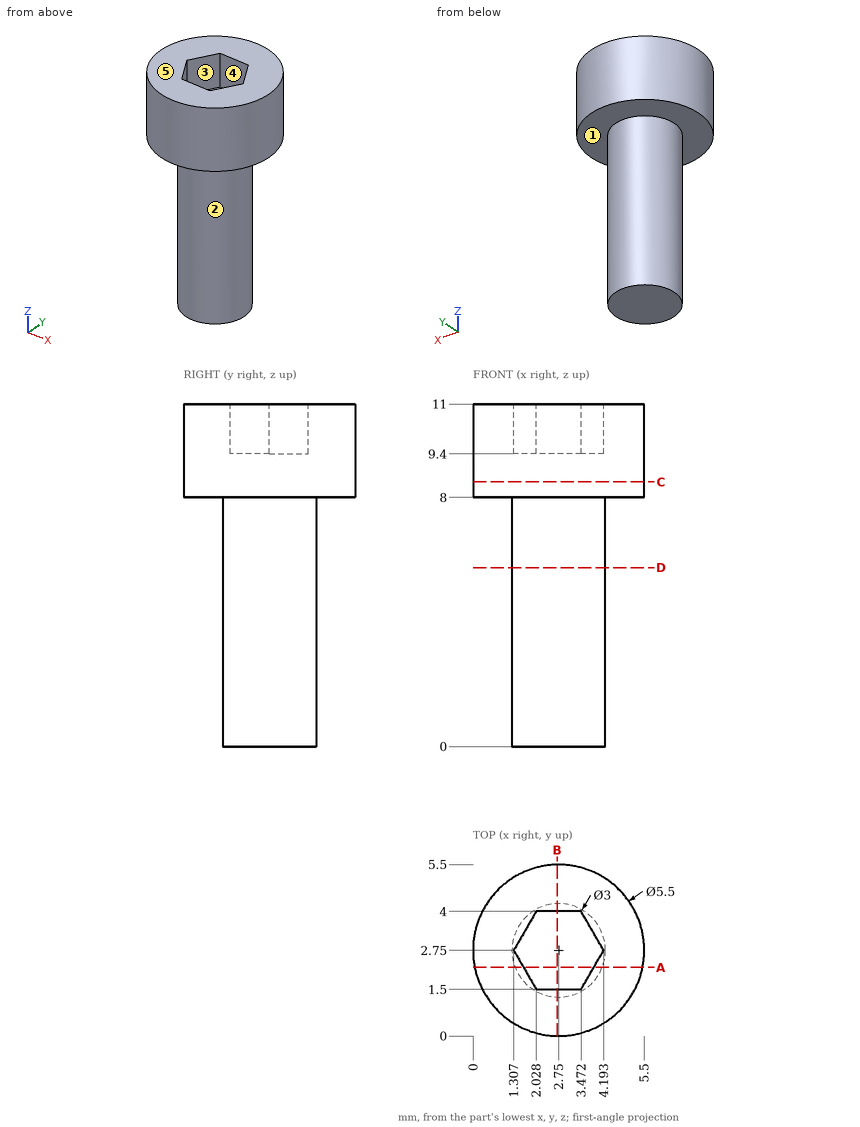
Verification items for this drawing (mm, ordinates from the low corner). A direction names the side the tool comes from. Coordinates: 2 decimals unless noted, no trailing zeros. Order: outer loops, then holes, each group sorted by start corner. A loop starts at its lowest first (then second) coordinate and runs counter-clockwise, first axis right, second up.
Q1. Sectioned sample at A-A on y = 2.2. Record the cut outline in (x, z) (1 decimal).
Reply:
outline: (0.1, 8) - (1.4, 8) - (1.4, 0) - (4.1, 0) - (4.1, 8) - (5.4, 8) - (5.4, 11) - (3.9, 11) - (3.9, 9.4) - (1.6, 9.4) - (1.6, 11) - (0.1, 11) - close
Q2. Tool access check on the marked faces 4 and 5. Record the directions out of +Z, -Z, +X, -X, +Y, -Y that give a thin tool (end or side, any length) a straight path to the whole face; none if there is none.
Reply:
face 4: +Z
face 5: +Z, +X, -X, +Y, -Y
Q3. Sectioned sample at B-B on x = 2.7. Record the cut outline in (y, z).
Reply:
outline: (0, 8) - (1.25, 8) - (1.25, 0) - (4.25, 0) - (4.25, 8) - (5.5, 8) - (5.5, 11) - (4, 11) - (4, 9.4) - (1.5, 9.4) - (1.5, 11) - (0, 11) - close
Q4. Thickness scan on probe 1 along X at (y, z) = (2.65, 8.25); probe 2 along Z at (x, y) = (3.1, 4.4); probe 3 along Z at (x, y) = (2.5, 2.85). Record the ranges inside material, lowest first.
Reply:
probe 1: x = 0 to 5.5
probe 2: z = 8 to 11
probe 3: z = 0 to 9.4
Q5. Sectioned sample at D-D on z = 5.75. Record the cut outline in (x, y).
Reply:
outline: circle Ø3 at (2.75, 2.75)
Q6. Sectioned sample at C-C on z = 8.5. Record the cut outline in (x, y).
Reply:
outline: circle Ø5.5 at (2.75, 2.75)
Q7. Depth check by flat-ended pin: pin 1 Ø2 at (y, z) = (4.5, 2.5) entering from -X; pin 2 Ø0.8 at (x, y) = (3, 2.5) entering from +Z; pin 3 Ø1 at (y, z) = (1, 9.5) entering from -X. Enter the tip coordinate at first touch or a pass-through.
Reply:
pin 1: stops at x = 1.45
pin 2: stops at z = 9.4
pin 3: stops at x = 0.3
Q8. Draft check along X on the marked faces 1, 2 and 3. Enter one of: released by +X, released by -X, zero draft, split by the parting line, or undercut.
Reply:
face 1: zero draft
face 2: split by the parting line
face 3: undercut
